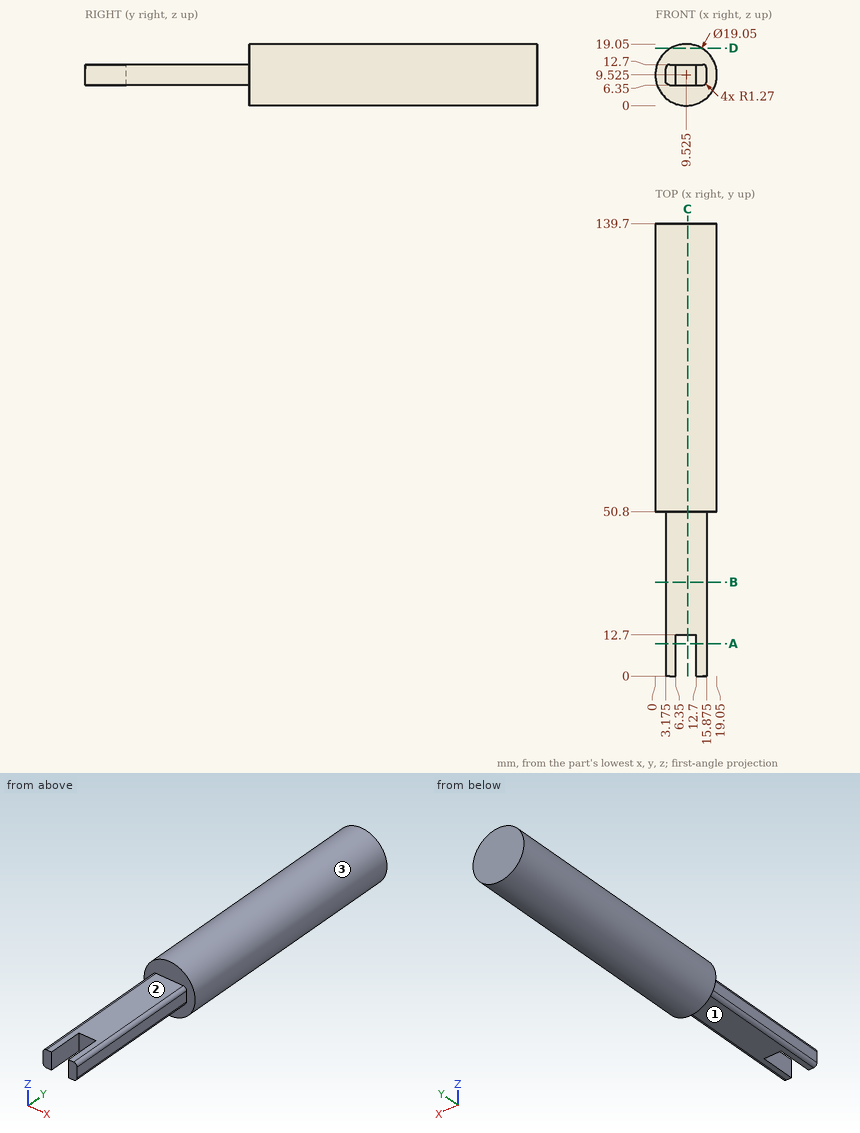
Part print with two shaded views. Sizes in mm from the minimum x, y, z corner. A direction names the side the tool comes from. Round coordinates to 2 decimals unless told otherwise and drop trailing zeros. Order: outer loops, then holes, each group sorted by start corner. A loop starts at its lowest first (then second) coordinate and runs counter-clockwise, first axis right, second up. Notation, with made-up numbers: M 88,-17 L 140,-17 A21 ccw 140,18 Z; hole C -21.5,-1.75 d6. An arc over 180 degrees is marked long. Answer in a Markdown table with one row per item. Add a question column.
Q1. Wall check: L1, parallel to Z at x = 13.5, y = 41; L2, parallel to Y at x = 14.5, z = 4.75; L3, parallel to X at y = 26.5, z = 11.5. Give the ranges that are in metal, low to high. Write a range as from..to.
Q2. Cut at C-C on x = 10. Give the cut face in (y, z), and give its area (3 significant figures).
Q3. Cut at D-D on z = 17.75. Give the cut face in (x, y), and give its area (3 significant figures).
Q4. Pin check, flat tips, straight feed: pin 1 (4 mm diameter, centred on y = 16, z = 10, fed in from -X) (3 decimals); pin 2 (1.5 mm diameter, centred on y = 88.5, z = 12, fed in from +X); pin 3 (1 mm diameter, centred on y = 64, z = 7, fed in from -X). Stop position of each tip, or through.
Q5. Cut at A-A on y = 10. Give the cut face in (x, z) (3 decimals).
Q6. 3-axis set-ups, long thin cutter, end or side, ignore diameter. For the marked faces 1, 2 and 3: which of +Z, -Z, +X, -X, +Y, -Y reach the whole face in a straight line?
Q7. Cut at B-B on y = 29. Give the cut face in (x, z) (3 decimals), and give its area (3 significant figures).
Established:
| question | item | result |
|---|---|---|
| 1 | L1 | z = 6.35..12.7 |
| 1 | L2 | y = 50.8..139.7 |
| 1 | L3 | x = 3.18..15.87 |
| 2 | outline | M 12.7,6.35 L 50.8,6.35 L 50.8,0.01 L 139.7,0.01 L 139.7,19.04 L 50.8,19.04 L 50.8,12.7 L 12.7,12.7 Z |
| 2 | area | 1,930 mm2 |
| 3 | outline | M 4.72,50.8 L 14.33,50.8 L 14.33,139.7 L 4.72,139.7 Z |
| 3 | area | 854 mm2 |
| 4 | pin 1 | stops at x = 3.175 |
| 4 | pin 2 | stops at x = 18.89 |
| 4 | pin 3 | stops at x = 0.22 |
| 5 | outline | M 3.175,7.62 A1.27 ccw 4.445,6.35 L 6.35,6.35 L 6.35,12.7 L 4.445,12.7 A1.27 ccw 3.175,11.43 Z; M 12.7,6.35 L 14.605,6.35 A1.27 ccw 15.875,7.62 L 15.875,11.43 A1.27 ccw 14.605,12.7 L 12.7,12.7 Z |
| 6 | face 1 | -Z, +X, -X, -Y |
| 6 | face 2 | +Z, +X, -X, -Y |
| 6 | face 3 | +Y, -Y |
| 7 | outline | M 3.175,7.62 A1.27 ccw 4.445,6.35 L 14.605,6.35 A1.27 ccw 15.875,7.62 L 15.875,11.43 A1.27 ccw 14.605,12.7 L 4.445,12.7 A1.27 ccw 3.175,11.43 Z |
| 7 | area | 79.3 mm2 |
